Here's how the part is built. I have some questions about the finished solid (model axes, mm). Coordinates: 2 decimals unless noted, no trailing zeros. Write each loop counter-clockwise with the first axis right and the second up, starting at its lowest first coordinate (ties: lowest second). Pieces come first, ordered by that corner, then holes.
Solid Edge part; units mm, degrees
sketch "Sketch1" plane through (0, 0, 0) normal (-1, 0, 0) x (0, -1, 0)
  line L0 (0, 0) -> (207.45, 0)
  line L1 (207.45, 0) -> (207.45, 214.47)
  line L2 (207.45, 214.47) -> (0, 214.47)
  line L3 (0, 214.47) -> (0, 0)
extrude "Protrusion1" add sketch "Sketch1" against normal blind 3
sketch "Sketch2" plane through (0, -103.725, 107.235) normal (-1, 0, 0) x (0, 1, 0)
  line L0 (-83.975, -28.235) -> (114.48, -28.235)
  line L1 (114.48, -28.235) -> (114.48, -31.235)
  line L2 (-83.975, -31.235) -> (114.48, -31.235)
  line L3 (-83.975, -28.235) -> (-83.975, -31.235)
  line L4 (-83.975, 11.765) -> (114.48, 11.765)
  line L5 (114.48, 11.765) -> (114.48, 14.765)
  line L6 (-83.975, 14.765) -> (114.48, 14.765)
  line L7 (-83.975, 11.765) -> (-83.975, 14.765)
  line L8 (-83.975, 57.765) -> (114.48, 57.765)
  line L9 (114.48, 57.765) -> (114.48, 54.765)
  line L10 (-83.975, 54.765) -> (114.48, 54.765)
  line L11 (-83.975, 57.765) -> (-83.975, 54.765)
  line L12 (-83.975, -74.235) -> (114.48, -74.235)
  line L13 (114.48, -74.235) -> (114.48, -71.235)
  line L14 (-83.975, -71.235) -> (114.48, -71.235)
  line L15 (-83.975, -74.235) -> (-83.975, -71.235)
  line L16 (-83.975, -104.235) -> (114.48, -104.235)
  line L17 (114.48, -104.235) -> (114.48, -107.235)
  line L18 (-83.975, -107.235) -> (114.48, -107.235)
  line L19 (-83.975, -104.235) -> (-83.975, -107.235)
  dimension "D1" = 114.48
  dimension "D2" = 83.975
  dimension "D3" = 114.48
  dimension "D4" = 83.975
extrude "Cutout1" cut sketch "Sketch2" against normal blind 10
sketch "Sketch3" plane through (0, -103.725, 107.235) normal (-1, 0, 0) x (0, 1, 0)
  line L0 (-118.847, 97.765) -> (179.5114, 97.765)
  line L1 (191.0928, 110.2989) -> (179.5114, 97.765)
  line L2 (-118.847, 116.9168) -> (191.0928, 110.2989)
  line L3 (-118.847, 97.765) -> (-118.847, 116.9168)
extrude "Cutout2" cut sketch "Sketch3" against normal blind 37
sketch "Sketch4" plane through (0, -103.725, 111.97) normal (-1, 0, 0) x (0, 1, 0)
  line L0 (-103.725, 102.5) -> (-103.725, -102.5)
  line L1 (-103.725, -102.5) -> (83.725, -102.5)
  line L2 (83.725, -102.5) -> (83.725, -99.5)
  line L3 (83.725, -99.5) -> (103.725, -99.5)
  line L4 (103.725, -99.5) -> (103.725, -69.5)
  line L5 (83.725, -69.5) -> (103.725, -69.5)
  line L6 (83.725, -66.5) -> (83.725, -69.5)
  line L7 (83.725, -66.5) -> (103.725, -66.5)
  line L8 (103.725, -66.5) -> (103.725, -26.5)
  line L9 (83.725, -26.5) -> (103.725, -26.5)
  line L10 (83.725, -23.5) -> (83.725, -26.5)
  line L11 (83.725, -23.5) -> (103.725, -23.5)
  line L12 (103.725, -23.5) -> (103.725, 16.5)
  line L13 (83.725, 16.5) -> (103.725, 16.5)
  line L14 (83.725, 19.5) -> (83.725, 16.5)
  line L15 (83.725, 19.5) -> (103.725, 19.5)
  line L16 (103.725, 19.5) -> (103.725, 59.5)
  line L17 (83.725, 59.5) -> (103.725, 59.5)
  line L18 (83.725, 62.5) -> (83.725, 59.5)
  line L19 (83.725, 62.5) -> (103.725, 62.5)
  line L20 (103.725, 62.5) -> (103.725, 102.5)
  line L21 (32.3413, 102.5) -> (103.725, 102.5)
  line L22 (-103.725, 102.5) -> (32.3413, 102.5)
  dimension "D1" = 103.725
extrude "Protrusion2" add sketch "Sketch4" along normal blind 3
sketch "Sketch5" plane through (0, -113.725, 214.47) normal (0, 0, 1) x (0, 1, 0)
  line L0 (-93.725, -3) -> (113.725, -3)
  line L1 (113.725, -3) -> (113.725, 3)
  line L2 (113.725, 3) -> (-93.725, 3)
  line L3 (-93.725, 3) -> (-93.725, -3)
extrude "Protrusion3" add sketch "Sketch5" along normal blind 15
sketch "Sketch6" plane through (-3, -103.725, 111.8236) normal (-1, 0, 0) x (0, 1, 0)
  circle A0 centre (93.725, 92.6464) radius 2
  circle A1 centre (16.725, 92.6464) radius 2
  circle A2 centre (-16.725, 92.6464) radius 2
  circle A3 centre (-93.725, -107.9393) radius 2
  circle A4 centre (93.725, -107.9393) radius 2
  circle A5 centre (16.725, -107.9393) radius 2
  circle A6 centre (-16.725, -107.9393) radius 2
  circle A7 centre (-93.725, 92.6464) radius 2
  dimension "D1" = 93.725
  dimension "D2" = 93.725
extrude "Cutout3" cut sketch "Sketch6" against normal blind 10
sketch "Sketch7" plane through (0, -103.725, 229.47) normal (0, 0, 1) x (0, 1, 0)
  line L0 (-86.2619, 0) -> (-115.3515, 0)
  line L1 (-115.3515, 0) -> (-115.3515, -14.0973)
  line L2 (-115.3515, -14.0973) -> (121.3932, -14.0973)
  line L3 (121.3932, -14.0973) -> (121.3932, 0)
  line L4 (121.3932, 0) -> (-86.2619, 0)
extrude "Cutout4" cut sketch "Sketch7" against normal blind 456
sketch "Sketch8" plane through (0, -103.725, 119.47) normal (1, 0, 0) x (0, -1, 0)
  line L0 (-83.725, 67) -> (-63.725, 67)
  line L1 (-63.725, 67) -> (-63.725, 70)
  line L2 (-63.725, 70) -> (-83.725, 70)
  line L3 (-83.725, 70) -> (-83.725, 67)
  line L4 (-83.725, 24) -> (-63.725, 24)
  line L5 (-63.725, 24) -> (-63.725, 27)
  line L6 (-63.725, 27) -> (-83.725, 27)
  line L7 (-83.725, 27) -> (-83.725, 24)
  line L8 (-83.725, -19) -> (-63.725, -19)
  line L9 (-63.725, -19) -> (-63.725, -16)
  line L10 (-63.725, -16) -> (-83.725, -16)
  line L11 (-83.725, -16) -> (-83.725, -19)
  line L12 (-83.725, -62) -> (-63.725, -62)
  line L13 (-63.725, -62) -> (-63.725, -59)
  line L14 (-63.725, -59) -> (-83.725, -59)
  line L15 (-83.725, -59) -> (-83.725, -62)
  line L16 (-83.725, -95) -> (-63.725, -95)
  line L17 (-63.725, -95) -> (-63.725, -92)
  line L18 (-63.725, -92) -> (-83.725, -92)
  line L19 (-83.725, -92) -> (-83.725, -95)
extrude "ExtrudedCutout_42" cut sketch "Sketch8" against normal blind 4
sketch "Sketch9" plane through (0, -103.725, 119.47) normal (1, 0, 0) x (0, 1, 0)
  line L0 (96.275, -147.6514) -> (96.275, 128.9829)
  line L1 (132.0943, 114.84) -> (96.275, 128.9829)
  line L2 (169.9971, 15.2743) -> (132.0943, 114.84)
  line L3 (96.275, -147.6514) -> (169.9971, 15.2743)
extrude "ExtrudedCutout_43" cut sketch "Sketch9" against normal blind 148
1. I want a section at A-A (y = -34). List the corners of the cut face in (x, z) for me, then the cut area to 3 significant figures.
2. If I drill on line 1 (Z direction, x = -0.75, y = -87); line 2 (Y direction, x = -1.5, z = 136.5); line 3 (Y direction, x = -2.3, z = 219), over which ranges is the centre line in solid material (lowest first)?
3. For pin 1 Ø0.9 at (x, z) = (-1, 136.5) entering from +Y, with a flat end and sliding along its axis, tell me the tip position at first contact or that it passes through.
Response values:
1. outline: (-3, 9.47) - (0, 9.47) - (0, 49.47) - (-3, 49.47) - close; (-3, 52.47) - (0, 52.47) - (0, 92.47) - (-3, 92.47) - close; (-3, 95.47) - (0, 95.47) - (0, 135.47) - (-3, 135.47) - close; (-3, 138.47) - (0, 138.47) - (0, 178.47) - (-3, 178.47) - close; (-3, 181.47) - (0, 181.47) - (0, 211.47) - (-3, 211.47) - close; (-3, 214.47) - (0, 214.47) - (0, 229.47) - (-3, 229.47) - close
1. area: 615 mm2
2. line 1: z = 9.47 to 17.18, 21.18 to 217.76, 221.76 to 229.47
2. line 2: y = -207.45 to -40
2. line 3: y = -207.45 to -199.3, -195.6 to -122.3, -118.6 to -88.85, -85.15 to -11.85, -8.15 to -7.45
3. pin 1: stops at y = -40
